from build123d import *

# Parameters (mm, degrees)
PAD_DEPTH = 10
FILLET_R  = 1


with BuildPart() as part:
    # Sketch → Pad (new body)
    with BuildSketch(Plane.XZ):
        Polygon((-3, 0), (-3, 3), (-3.25, 3.433013), (-1, 3.433013), (-2.249514, 0), (2.249514, 0), (1, 3.433013), (3.25, 3.433013), (3, 3), (3, 0), (6, 0), (6, -0.6), (-6, -0.6), (-6, 0), align=None)
    extrude(amount=PAD_DEPTH)

    # Fillet
    fillet_edges = [part.edges().sort_by_distance(p)[0] for p in [
        (-2.249514, -5, 0),
        (2.249514, -5, 0),
    ]]
    fillet(fillet_edges, radius=FILLET_R)


solid = part.part
Part model, mm, in its own coordinate system. A direction names the side the tool comes from. Give positions to 0.01 mm unless a question says otherwise; leave off trailing zeros. Write each loop counter-clockwise with the first axis right and the second up, starting at its lowest first coordinate (ties: lowest second). Pieces come first, ordered by that corner, then holes.
1) Cut at D-D on x = -4. Write the cut outline in (y, z), then the cut area to 3 significant figures.
Resolved:
outline: (-10, -0.6) - (0, -0.6) - (0, 0) - (-10, 0) - close
area: 6.00 mm2
2) Which spindle directions (+Z, -Z, +X, -X, +Y, -Y) get a long thin tool onto all of the face, cutting with end or side? Do faces 5 (the face through (3, -5, 2)), 6 (the face through (2, -5, 3.433)), 7 (the face through (-1.65, -5.07, 0.44)), 8 (the face through (0, -5, -0.6)), 9 (the face through (0, -5, 0)). Say none if no direction does.
Resolved:
face 5: +X, +Y, -Y
face 6: +Z, +X, -X, +Y, -Y
face 7: +Y, -Y
face 8: -Z, +X, -X, +Y, -Y
face 9: +Z, +Y, -Y
3) Probe L1, parallel to Z at x = 5, y = -9.5; L2, parallel to X at y = -3.5, z = 2.7; L3, parallel to X at y = -5.5, z = 1.75. List the from-to ranges inside material, lowest first.
Resolved:
L1: z = -0.6 to 0
L2: x = -3 to -1.27, 1.27 to 3
L3: x = -3 to -1.61, 1.61 to 3
4) Cut at B-B on z = 0.65. Write the cut outline in (x, y).
Resolved:
outline: (-3, -10) - (-1.76, -10) - (-1.76, 0) - (-3, 0) - close; (1.76, -10) - (3, -10) - (3, 0) - (1.76, 0) - close
5) Cut at C-C on x = 1.25. Write the cut outline in (y, z), then the cut area to 3 significant figures.
Resolved:
outline: (-10, -0.6) - (0, -0.6) - (0, 0.1) - (-10, 0.1) - close; (-10, 2.75) - (0, 2.75) - (0, 3.43) - (-10, 3.43) - close
area: 13.8 mm2
6) Two-plate mould, pull along Z, no slides. Class faces 1 (the face through (-3, -5, 1)), 2 (the face through (1.633, -5.07, 0.415)), 3 (the face through (0.1, 0, -0.3)), 4 (the face through (-2, -5, 3.433)): released by +Z, released by -Z, zero draft, split by the parting line, or undercut.
Resolved:
face 1: undercut
face 2: undercut
face 3: zero draft
face 4: released by +Z
7) Pin check, flat tips, straight feed: pin 1 (0.9 mm diameter, centred on x = -4.5, y = -6.5, fed in from +Z); pin 2 (0.9 mm diameter, centred on y = -6.5, z = 1, fed in from -X); pin 3 (1.5 mm diameter, centred on y = -2.5, z = 1, fed in from +X). Stop position of each tip, or through.
Resolved:
pin 1: stops at z = 0
pin 2: stops at x = -3
pin 3: stops at x = 3
8) Cut at A-A on y = -5. Write the cut outline in (x, z), then the cut area to 3 significant figures.
Resolved:
outline: (-6, -0.6) - (6, -0.6) - (6, 0) - (3, 0) - (3, 3) - (3.25, 3.43) - (1, 3.43) - (1.76, 1.34) arc R1 cw to (0.82, 0) - (-0.82, 0) arc R1 cw to (-1.76, 1.34) - (-1, 3.43) - (-3.25, 3.43) - (-3, 3) - (-3, 0) - (-6, 0) - close
area: 17.7 mm2
